Could you check a few things on this drawing? It's one solid part, dimensions in mm from its lowest x, y, z. A direction names the side the tool comes from. Round coordinates to 2 decimals unless told otherwise and drop trailing zeros. Loops run counter-clockwise (first coordinate to the right, second up) from the corner with the lowest first, then second, coordinate; pieces in that order, holes last. Notation, with made-up numbers: (69.5, -5.75) -> (127.5, -5.75) arc R21 cw to (127.5, 19.25) -> close; hole circle Ø7 at (45.5, 14.5). An arc over 180 degrees is marked (long way). Use one line per item in the form item = value. Start each with the question number.
Item 1: I'm going to push flat-ended pins straight in: pin 1 Ø1.8 at (y, z) = (6, 13.5) entering from -X; pin 2 Ø4 at (y, z) = (4, 34.5) entering from -X; pin 3 Ø1.5 at (x, z) = (16.5, 10) entering from -Y; pin 4 Ø5 at (x, z) = (11, 43) entering from -Y. Where does each tip first touch, or does it pass through?
Item 2: If we section it at A-A (x = 19): Write out the boundary of the cut face in (y, z), then the cut area to 3 significant figures.
Item 3: Thinking about a two-plate mould opening in X: for the marked faces 3, 4, 5 and 6, which applies, released by +X, released by -X, zero draft, split by the parting line, or undercut?
Item 4: If we section it at C-C (x = 26): Write out the boundary of the cut face in (y, z).
Item 5: If we section it at D-D (z = 47): Write out the boundary of the cut face in (x, y).
Item 6: If I drill on L1, parallel to X at y = 5.75, z = 43; L2, parallel to X at y = 3, z = 20.5; L3, parallel to X at y = 1.5, z = 43.5, over which ranges is the centre line in solid material (lowest first)? Write a range as [from, to].
Item 7: If we section it at B-B (y = 7): Write out the boundary of the cut face in (x, z).
Item 8: For the marked faces 1 and 2, which set-ups out of +Z, -Z, +X, -X, +Y, -Y let a thin tool reach every point of the face, with its end or its side?
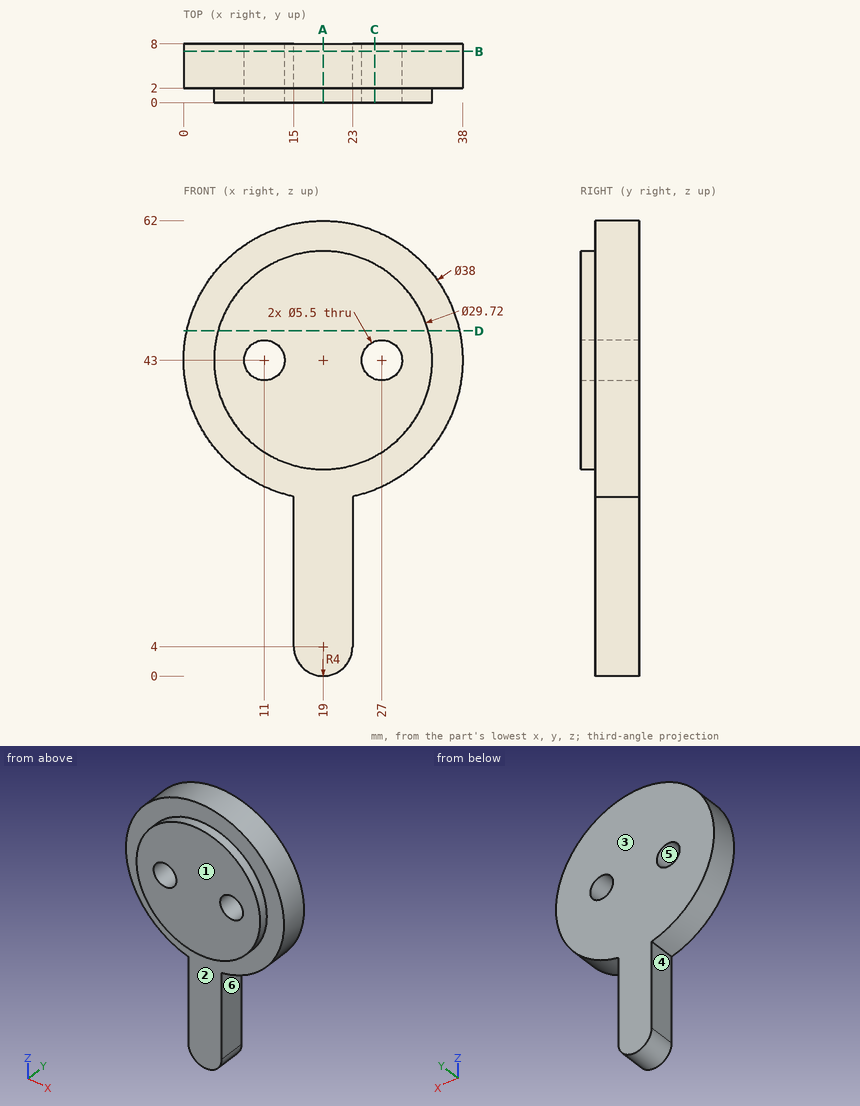
Values found:
q1.pin_1 = 15
q1.pin_2 = 1.15
q1.pin_3 = 2
q1.pin_4 = through
q2.outline = (0, 28.14) -> (2, 28.14) -> (2, 0) -> (8, 0) -> (8, 62) -> (2, 62) -> (2, 57.86) -> (0, 57.86) -> close
q2.area = 431 mm2
q3.face_3 = zero draft
q3.face_4 = released by -X
q3.face_5 = undercut
q3.face_6 = released by +X
q4.outline = (0, 29.89) -> (2, 29.89) -> (2, 25.34) -> (8, 25.34) -> (8, 40.44) -> (0, 40.44) -> close; (0, 45.56) -> (8, 45.56) -> (8, 60.66) -> (2, 60.66) -> (2, 56.11) -> (0, 56.11) -> close
q5.outline = (0.43, 2) -> (4.69, 2) -> (4.69, 0) -> (33.31, 0) -> (33.31, 2) -> (37.57, 2) -> (37.57, 8) -> (0.43, 8) -> close
q6.L1 = [0, 8.25], [13.75, 24.25], [29.75, 38]
q6.L2 = [15, 23]
q6.L3 = [4.15, 8.3], [13.7, 24.3], [29.7, 33.85]
q7.outline = (15, 4) arc R4 ccw to (23, 4) -> (23, 24.43) arc R19 ccw (long way) to (15, 24.43) -> close; hole circle Ø5.5 at (11, 43); hole circle Ø5.5 at (27, 43)
q8.face_1 = +Z, -Z, +X, -X, -Y
q8.face_2 = -Y
